Can you work these out from the model? Positions are in its coordinate system, mm. Face numbers are marked on the shaded views. A direction names the side the tool comes from. Round coordinates to 2 decimals unless told otherwise and drop trailing zeros. Write each loop counter-clockwise with the first axis right and the second up, starting at its lowest first coordinate (ties: lowest second). Pieces come first, ordered by that corner, then holes. Notation, with made-up numbers: (35.5, -14.5) - (60.5, -14.5) arc R6 cw to (60.5, -10.5) - close; hole circle Ø4 at (43, 36.25). An arc over 180 degrees is marked (long way). One line per item, written item: value. Start each with the question number.
(1) I'm going to push flat-ended pins straight in: pin 1 Ø3.5 at (y, z) = (-7, -0.5) entering from +X; pin 2 Ø2.5 at (y, z) = (-7.5, -0.5) entering from -X; pin 3 Ø3 at (y, z) = (11, 1.5) entering from +X. Where does each tip first touch, or does it pass through?
(2) If I drill on L1, parallel to X at y = -2.25, z = -0.25; L2, parallel to Y at x = 4.75, z = 0; L3, parallel to Y at x = -4.75, z = -1.5, over which ranges is the centre line in solid material (lowest first)? Write a range as from..to.
(3) I want a section at C-C on x = 2. List the corners of the cut face in (y, z) for me.
(4) I want a section at D-D on x = 4.75. List the corners of the cut face in (y, z) for me, plus the area to 3 significant figures.
(5) I want a section at B-B on z = -0.5. List the corners of the cut face in (x, y) for me.
(6) I want a section at A-A on y = -2.2. List the corners of the cut face in (x, z) for me.
(7) On a 3-axis mill with a long thin cutter (end or side, diameter ignored), from which of +Z, -Z, +X, -X, +Y, -Y can I reach the whole of each face in a straight line? I mean the marked faces 4, 5, 6, 7 and 8. Say none if no direction works.
(8) Thinking about a two-plate mould opening in X: for the marked faces 1, 2 and 3, which applies, +X half, -X half, draft (parallel to the pull), parting line (faces both ways), or undercut?
from build123d import *

# Parameters (mm, degrees)
SKETCH1_W           = 20
SKETCH1_H           = 10.2
SKETCH1_R           = 1.25
BOSS_EXTRUDE1_DEPTH = 3.2
BOSS_EXTRUDE2_DEPTH = 2
SKETCH3_W           = 3.3
SKETCH3_H           = 3.5
BOSS_EXTRUDE3_DEPTH = 0.25
BOSS_EXTRUDE4_START = 8.8
SKETCH3_2_W         = 3.3
SKETCH3_2_H         = 3.5
BOSS_EXTRUDE4_DEPTH = 0.25
BOSS_EXTRUDE5_START = -7.3
SKETCH3_3_W         = 3.3
SKETCH3_3_H         = 3.5
BOSS_EXTRUDE5_DEPTH = 0.25


with BuildPart() as part:
    # Sketch1 → Boss-Extrude1 (new, symmetric)
    with BuildSketch(Plane.XY):
        Rectangle(SKETCH1_W, SKETCH1_H)
        with Locations((-4.75, -2.2)):
            Circle(SKETCH1_R, mode=Mode.SUBTRACT)
        with Locations((4.75, -2.2)):
            Circle(SKETCH1_R, mode=Mode.SUBTRACT)
    extrude(amount=BOSS_EXTRUDE1_DEPTH, both=True)

    # Sketch2 → Boss-Extrude2 (add, symmetric)
    with BuildSketch(Plane.XY):
        with BuildLine():
            Line((7.25, 5.1), (6.85, 5.1))
            Line((6.85, 5.1), (6.85, 5.749556363))
            Line((6.85, 5.749556363), (-11.637609905, 8.201949589))
            Line((-11.637609905, 8.201949589), (-11.335934652, 10.476158449))
            ThreePointArc((-11.335934652, 10.476158449), (-8.965116404, 13.9), (-7.56893257, 9.976463224))
            Line((-7.56893257, 9.976463224), (-7.818008326, 8.098780899))
            Line((-7.818008326, 8.098780899), (7.25, 6.1))
            Line((7.25, 6.1), (7.25, 5.1))
        make_face()
    extrude(amount=BOSS_EXTRUDE2_DEPTH, both=True)

    # Sketch3 → Boss-Extrude3 (add, symmetric)
    with BuildSketch(Plane(origin=(0, 0, 0), x_dir=(0, 0, -1), z_dir=(1, 0, 0))):
        with Locations((0, -6.85)):
            Rectangle(SKETCH3_W, SKETCH3_H)
    extrude(amount=BOSS_EXTRUDE3_DEPTH, both=True)

    # Sketch3<2> → Boss-Extrude4 (add, symmetric)
    with BuildSketch(Plane(origin=(0, 0, 0), x_dir=(0, 0, -1), z_dir=(1, 0, 0)).offset(BOSS_EXTRUDE4_START)):
        with Locations((0, -6.85)):
            Rectangle(SKETCH3_2_W, SKETCH3_2_H)
    extrude(amount=BOSS_EXTRUDE4_DEPTH, both=True)

    # Sketch3<3> → Boss-Extrude5 (add, symmetric)
    with BuildSketch(Plane(origin=(0, 0, 0), x_dir=(0, 0, -1), z_dir=(1, 0, 0)).offset(BOSS_EXTRUDE5_START)):
        with Locations((0, -6.85)):
            Rectangle(SKETCH3_3_W, SKETCH3_3_H)
    extrude(amount=BOSS_EXTRUDE5_DEPTH, both=True)


solid = part.part
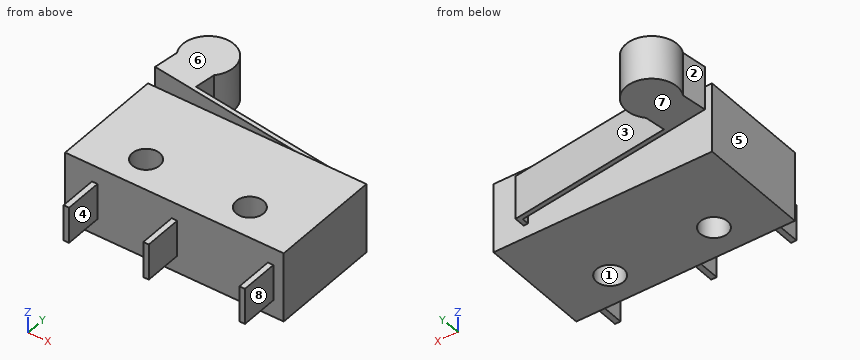
Established:
1. pin 1: x = 9.05
1. pin 2: x = -7.55
1. pin 3: x = -6.93
2. L1: -10..-6, -3.5..3.5, 6..10
2. L2: -5.1..-3.45, -0.95..5.1, 6.03..6.43
2. L3: -5.1..-3.45, -0.95..5.1, 7.29..7.69
3. outline: (-5.1, -3.2) - (5.1, -3.2) - (5.1, 3.2) - (-5.1, 3.2) - close; (6.39, -2) - (6.8, -2) - (6.8, 2) - (6.39, 2) - close
4. outline: (-5.1, -3.2) - (-3.45, -3.2) - (-3.45, 3.2) - (-5.1, 3.2) - close; (-0.95, -3.2) - (5.1, -3.2) - (5.1, 3.2) - (-0.95, 3.2) - close; (6.03, -2) - (6.43, -2) - (6.43, 2) - (6.03, 2) - close
4. area: 50.9 mm2
5. outline: (-11.64, 8.2) - (6.85, 5.75) - (6.85, 5.1) - (-10, 5.1) - (-10, -5.1) - (-7.55, -5.1) - (-7.55, -8.6) - (-7.05, -8.6) - (-7.05, -5.1) - (-0.25, -5.1) - (-0.25, -8.6) - (0.25, -8.6) - (0.25, -5.1) - (8.55, -5.1) - (8.55, -8.6) - (9.05, -8.6) - (9.05, -5.1) - (10, -5.1) - (10, 5.1) - (7.25, 5.1) - (7.25, 6.1) - (-7.82, 8.1) - (-7.57, 9.98) arc R2.34 ccw (long way) to (-11.34, 10.48) - close; hole circle Ø2.5 at (-4.75, -2.2); hole circle Ø2.5 at (4.75, -2.2)
6. outline: (-10, -3.2) - (-6, -3.2) - (-6, 3.2) - (-10, 3.2) - close; (-3.5, -3.2) - (3.5, -3.2) - (3.5, 3.2) - (-3.5, 3.2) - close; (6, -3.2) - (10, -3.2) - (10, 3.2) - (6, 3.2) - close
7. face 4: +Z, -Z, -Y
7. face 5: +Z, -Z, -X, -Y
7. face 6: +Z, +X, -X, +Y
7. face 7: -Z, +X, -X, +Y
7. face 8: +Z, -Z, +X, -Y
8. face 1: undercut
8. face 2: -X half
8. face 3: +X half
